The listing builds one solid part. Answer for the finished solid, in the listing's coordinates (mm). Face numbers are marked on the shaded views. Give positions to 0.01 mm unless a question says otherwise; leave off trailing zeros. Write each loop counter-clockwise with the first axis right and the second up, starting at its lowest first coordinate (ties: lowest second). Pieces come first, ordered by that corner, then holes. Notation, with made-up numbers: (53.5, 47) - (96.5, 47) arc R27 cw to (96.5, 73) - close; hole circle Ø4 at (0.25, 8). An arc over 180 degrees is marked (long way). One line per question, with ' | ' between items. Start each with the question number.
1. Given P1, Ø11, axis at y = 6, z = -7.5, coming from the +X side; P2, Ø6, axis at x = 7.5, z = -13, coming from the -Y side; P3, Ø5, axis at x = 4, z = 6, coming from the +Y side; P4, Ø5, axis at x = 19.5, y = -5.5, coming from the +Z side, each flat-ended and moving along its own axis, determine where each tip first touches the part or whether it passes through.
2. The mould has two halves that part along Y. Classify the marked faces 1, 2, 3 and 4: +Y half, -Y half, draft (parallel to the pull), parting line (faces both ways), or undercut.
3. A cutting plane is placed at A-A (x = 12). Determine the outline of the cut face in (y, z) (1 decimal).
4. Find the intervals of material crossed by L1, parallel to Y at x = 17, z = 0; L2, parallel to X at y = 17.5, z = -5.5; L3, parallel to Y at x = 8.5, z = -9.5, in increasing order. Write a range as from..to.
```python
from build123d import *

# Parameters (mm, degrees)
BASENUT_DEPTH = 18.288


# Read off the part's stored shape, not the designer's step: ThreadSchematic
with BuildPart() as part:
    # BaseNutSke → BaseNut (new body)
    with BuildSketch(Plane(origin=(0, 0, 0), x_dir=(0, 0, -1), z_dir=(1, 0, 0))):
        Polygon((18.25625, 10.540250852), (18.25625, -10.540250852), (0, -21.080501704), (-18.25625, -10.540250852), (-18.25625, 10.540250852), (0, 21.080501704), align=None)
    extrude(amount=BASENUT_DEPTH)

    # Sketch3 → Crown (revolve)
    with BuildSketch(Plane.XY, mode=Mode.PRIVATE) as crown_sk:
        with BuildLine():
            Line((39.37, 0), (0, 0))
            Line((0, 0), (0, 17.907))
            Line((0, 17.907), (19.111504465, 17.907))
            ThreePointArc((19.111504465, 17.907), (31.849674106, 13.489376766), (39.117596428, 2.1336))
            ThreePointArc((39.117596428, 2.1336), (39.306679868, 1.074238861), (39.37, 0))
        make_face()
    revolve(crown_sk.sketch.rotate(Axis((0, 0, 0), (1, 0, 0)), 90), axis=Axis((0, 0, 0), (1, 0, 0)))

    # Sketch4 → DoubleChamfer (revolve, cut)
    with BuildSketch(Plane.XY, mode=Mode.PRIVATE) as doublechamfer_sk:
        Polygon((0, 18.25625), (1.955420677, 25.553979317), (16.332934387, 25.553979317), (18.288, 18.25625), (30.988, 18.25625), (30.988, 43.65625), (-12.7, 43.65625), (-12.7, 18.25625), align=None)
    revolve(doublechamfer_sk.sketch.rotate(Axis((0, 0, 0), (1, 0, 0)), 90), axis=Axis((0, 0, 0), (1, 0, 0)), mode=Mode.SUBTRACT)

    # ThreadSchematic outline → ThreadSchematic (revolve, cut)
    with BuildSketch(Plane.YX):
        Polygon((11.1125, 0), (11.1125, 28.448), (0, 35.125063629), (0, 0), align=None)
    revolve(axis=Axis((0, 0, 0), (1, 0, 0)), mode=Mode.SUBTRACT)

    # EndChamferSketch → EndChamfer (revolve, cut)
    with BuildSketch(Plane.XY, mode=Mode.PRIVATE) as endchamfer_sk:
        Polygon((-0.0254, 12.7), (0.0254, 12.7), (1.248137414, 10.95375), (-0.0254, 10.95375), align=None)
    revolve(endchamfer_sk.sketch.rotate(Axis((0, 0, 0), (-1, 0, 0)), 270), axis=Axis((0, 0, 0), (-1, 0, 0)), mode=Mode.SUBTRACT)


solid = part.part
```
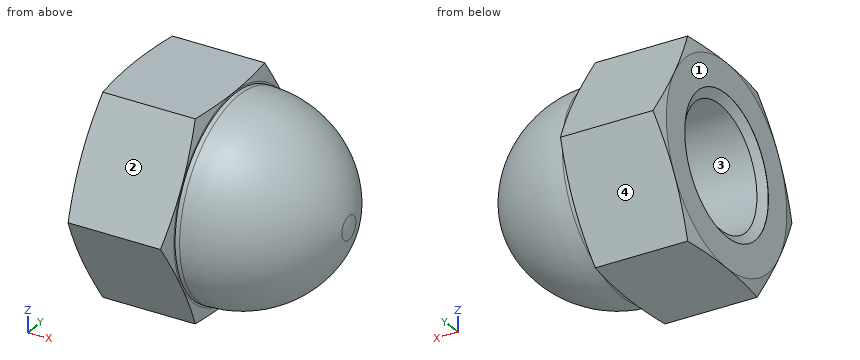
Determined:
1) P1: x = 38.54 | P2: y = -15.31 | P3: y = 19.06 | P4: z = 18.26
2) face 1: draft | face 2: -Y half | face 3: undercut | face 4: +Y half
3) outline: (-21.1, 0) - (-10.5, -18.3) - (10.5, -18.3) - (21.1, 0) - (10.5, 18.3) - (-10.5, 18.3) - close; hole circle Ø22.2 at (0, 0)
4) L1: -21.08..-11.11, 11.11..21.08 | L2: 0.02..18.26 | L3: -15.6..-5.77, 5.77..15.6
